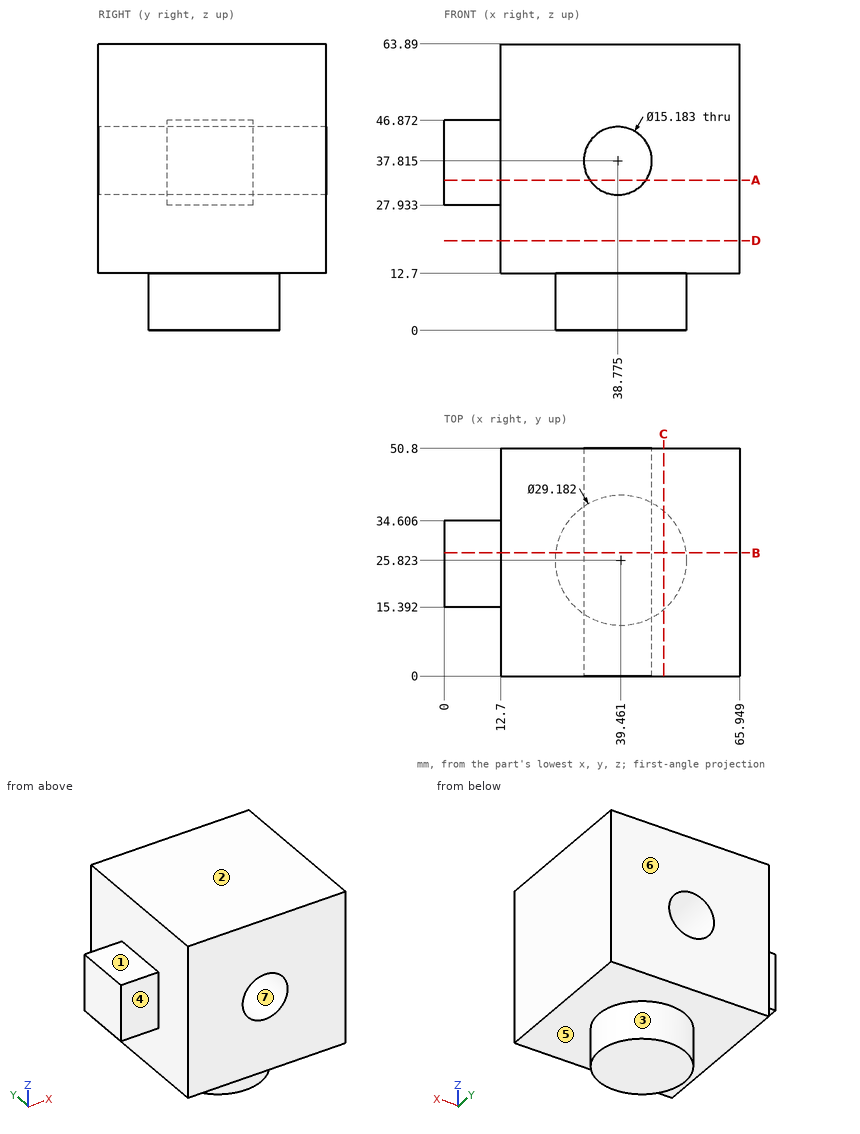
Answer from the drawing. Dimensions are ordinates in mm from the lowest x, y and z of the part. A direction names the side the tool comes from. Coordinates: 2 decimals unless noted, no trailing zeros. Loops run counter-clockwise (first coordinate to the right, second up) from the corner with the lowest first, then second, coordinate; pieces in that order, holes last.
1) Section D-D (z = 20) is taken. Give the vertices of the cut face in (x, y), plus the area to 4 significant figures.
Results:
outline: (12.7, 0) - (65.95, 0) - (65.95, 50.8) - (12.7, 50.8) - close
area: 2,705 mm2
2) Section A-A (z = 33.5) is taken. Give the vertices of the cut face in (x, y) (1 decimal), plus the area to 3 significant figures.
Results:
outline: (0, 15.4) - (12.7, 15.4) - (12.7, 0) - (32.5, 0) - (32.5, 50.8) - (12.7, 50.8) - (12.7, 34.6) - (0, 34.6) - close; (45, 0) - (65.9, 0) - (65.9, 50.8) - (45, 50.8) - close
area: 2,310 mm2
3) Section C-C (x = 49) is taken. Give the vertices of the cut face in (y, z) (1 decimal).
Results:
outline: (0, 12.7) - (14.8, 12.7) - (14.8, 0) - (36.9, 0) - (36.9, 12.7) - (50.8, 12.7) - (50.8, 63.9) - (0, 63.9) - close
4) Section B-B (y = 27.5) is taken. Give the vertices of the cut face in (x, z) (1 decimal), plus the area to 3 significant figures.
Results:
outline: (0, 27.9) - (12.7, 27.9) - (12.7, 12.7) - (25, 12.7) - (25, 0) - (54, 0) - (54, 12.7) - (65.9, 12.7) - (65.9, 63.9) - (12.7, 63.9) - (12.7, 46.9) - (0, 46.9) - close; hole circle Ø15.2 at (38.8, 37.8)
area: 3,150 mm2
5) Flat-ended cylindrical pins translate along their axes: pin 1 (6.5 mm diameter, centred on x = 4.5, z = 35.5, fed in from +Y); pin 2 (15 mm diameter, centred on x = 44, y = 22, fed in from -Z); pin 3 (10 mm diameter, centred on x = 7, y = 26, fed in from -Z); pin 4 (6.5 mm diameter, centred on x = 5.5, y = 25.5, fed in from +Z). Find the tip coordinate at first contact, or state that the pin passes through.
Results:
pin 1: stops at y = 34.61
pin 2: stops at z = 0
pin 3: stops at z = 27.93
pin 4: stops at z = 46.87
6) Consider probe 1 along Z at (x, y) = (33, 48) (1 decimal); probe 2 along Z at (x, y) = (63, 39); probe 3 along X at (y, z) = (33, 41.5). Determine where each line is inside the solid, lowest interval first.
Results:
probe 1: z = 12.7 to 32.9, 42.7 to 63.9
probe 2: z = 12.7 to 63.89
probe 3: x = 0 to 32.14, 45.41 to 65.95
7) For a pull along Z with two mould halves and no side action, classify the marked faces 5, 6 and 7 as +Z half, -Z half, draft (parallel to the pull), parting line (faces both ways), or undercut.
Results:
face 5: -Z half
face 6: draft
face 7: undercut
8) For the marked faces 1, 2, 3 and 4, determine the directions among +Z, -Z, +X, -X, +Y, -Y from which every point of the face is accessible in a straight line to the end or side of a thin tool.
Results:
face 1: +Z, -X, +Y, -Y
face 2: +Z, +X, -X, +Y, -Y
face 3: -Z
face 4: +Z, -Z, -X, -Y
